Autodesk Inventor part; units mm, degrees
ref_plane "YZ Plane" through (0, 0, 0) normal (1, 0, 0) x (0, 1, 0)
ref_plane "XZ Plane" through (0, 0, 0) normal (0, 1, 0) x (-1, 0, 0)
ref_plane "XY Plane" through (0, 0, 0) normal (0, 0, 1) x (1, 0, 0)
sketch "Sketch1" plane through (0, 0, 0) normal (0, 0, 1) x (1, 0, 0)
  line L0 (0, 0) -> (0, 1)
  line L1 (0, 1) -> (0, 15)
  line L2 (0, 15) -> (20, 15)
  line L3 (20, 15) -> (20, 10)
  line L4 (20, 10) -> (19, 10)
  line L5 (19, 10) -> (19, 14)
  line L6 (19, 14) -> (1, 14)
  line L7 (1, 14) -> (1, 0)
  line L8 (1, 0) -> (-101, 0)
  line L9 (-101, 0) -> (-101, 14)
  line L10 (-101, 14) -> (-119, 14)
  line L11 (-119, 14) -> (-119, 10)
  line L12 (-119, 10) -> (-120, 10)
  line L13 (-120, 10) -> (-120, 15)
  line L14 (-120, 15) -> (-100, 15)
  line L15 (-100, 15) -> (-100, 1)
  line L16 (-100, 1) -> (0, 1)
  dimension "d1" = 14
  dimension "d2" = 20
  dimension "d3" = 5
  dimension "d4" = 1
  dimension "d5" = 4
  dimension "d6" = 18
  dimension "d7" = 102
  dimension "d8" = 14
  dimension "d9" = 18
  dimension "d10" = 4
  dimension "d11" = 1
  dimension "d12" = 5
  dimension "d13" = 20
  dimension "d14" = 14
extrude "Extrusion1" add sketch "Sketch1" along normal blind 120
sketch "Sketch2" plane through (0, 15, 0) normal (0, 1, 0) x (1, 0, 0)
  circle A0 centre (10, -85) radius 5
  circle A1 centre (10, -35) radius 5
  circle A2 centre (-110, -35) radius 5
  circle A3 centre (-110, -85) radius 5
  line L0 (20, 0) -> (20, -120)
  line L1 (20, 0) -> (0, 0)
  line L2 (20, -120) -> (0, -120)
  line L3 (-120, 0) -> (-120, -120)
  dimension "d17" = 10
  dimension "d18" = 10
  dimension "d19" = 10
  dimension "d20" = 10
hole "Hole1" at (10, 15, 85) at (10, 15, 35) at (-110, 15, 35) at (-110, 15, 85) direction (0, -1, 0) diameter 10 end through all
properties part number "Pallet"
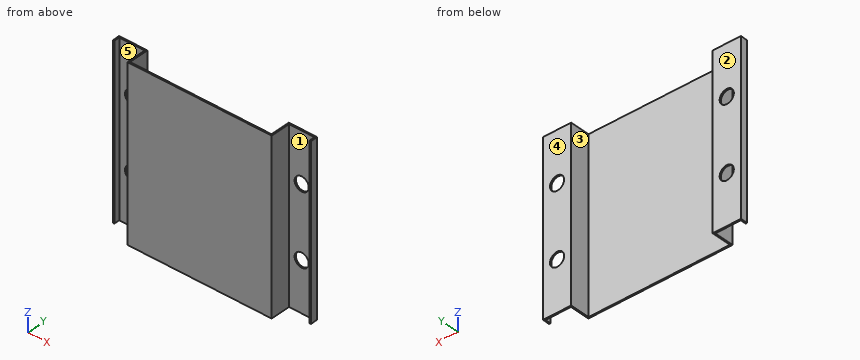
Check sheet for the modelled part. Datum: model origin and axes. Units: mm. Face numbers are marked on the shaded views. A direction names the side the tool comes from. Coordinates: 2 decimals unless noted, no trailing zeros. Loops run counter-clockwise (first coordinate to the right, second up) from the corner with the lowest first, then second, coordinate; pieces in that order, holes last.
1) Sectioned sample at C-C (x = 10). Record the boundary of the cut face in (y, z), and give its area (3 significant figures).
2) Release check for a two-part mould opening along X. For the marked faces 1 and 2 record: released by +X, released by -X, zero draft, split by the parting line, or undercut.
3) Sectioned sample at D-D (z = 12.5). Record the boundary of the cut face in (x, y), and give its area (3 significant figures).
4) Sectioned sample at A-A (y = 5.25). Record the boundary of the cut face in (x, z).
5) Gauge pin test, flat ends, axial feed: pin 1 (9 mm diameter, centred on x = 10, z = 35, fed in from -Y); pin 2 (3 mm diameter, centred on y = 4.5, z = 61.5, fed in from +X); pin 3 (0.8 mm diameter, centred on x = 19.5, z = 37, fed in from -Y); pin 4 (1.5 mm diameter, centred on y = 2.5, z = 12, fed in from -X). Record the tip position at first contact, or that the pin passes through.
6) Material ranges on probe 1 along Z at (x, y) = (-110, 14.5); probe 2 along X at (y, z) = (14.5, 85); probe 3 along X at (y, z) = (13.75, 5), recorded low to high.
7) Sectioned sample at B-B (z = 85). Record the boundary of the cut face in (x, y), and give its area (3 significant figures).
8) Access from +Z, -Z, +X, -X, +Y, -Y to the whole of each face (thin tool, end or side, straight path). Record for the marked faces 3, 4 and 5.
Check sheet entries:
1. outline: (14, 0) - (15, 0) - (15, 30) - (14, 30) - close; (14, 40) - (15, 40) - (15, 80) - (14, 80) - close; (14, 90) - (15, 90) - (15, 120) - (14, 120) - close
1. area: 100 mm2
2. face 1: undercut
2. face 2: zero draft
3. outline: (-120, 10) - (-119, 10) - (-119, 14) - (-101, 14) - (-101, 0) - (1, 0) - (1, 14) - (19, 14) - (19, 10) - (20, 10) - (20, 15) - (0, 15) - (0, 1) - (-100, 1) - (-100, 15) - (-120, 15) - close
3. area: 176 mm2
4. outline: (-101, 0) - (-100, 0) - (-100, 120) - (-101, 120) - close; (0, 0) - (1, 0) - (1, 120) - (0, 120) - close
5. pin 1: passes through
5. pin 2: stops at x = 1
5. pin 3: stops at y = 10
5. pin 4: stops at x = -101
6. probe 1: z = 0 to 30, 40 to 80, 90 to 120
6. probe 2: x = -120 to -115, -105 to -100, 0 to 5, 15 to 20
6. probe 3: x = -120 to -119, -101 to -100, 0 to 1, 19 to 20
7. outline: (-120, 10) - (-119, 10) - (-119, 14) - (-115, 14) - (-115, 15) - (-120, 15) - close; (-105, 14) - (-101, 14) - (-101, 0) - (1, 0) - (1, 14) - (5, 14) - (5, 15) - (0, 15) - (0, 1) - (-100, 1) - (-100, 15) - (-105, 15) - close; (15, 14) - (19, 14) - (19, 10) - (20, 10) - (20, 15) - (15, 15) - close
7. area: 156 mm2
8. face 3: +Z, -Z, +Y
8. face 4: +Z, -Z, +X, -X, +Y
8. face 5: +Z, -Z, -Y
